Source: CAD feature listing. Evaluate the final solid. Frame: model axes, mm. Face numbers are marked on the shaded views. A direction names the side the tool comes from. Give positions to 0.01 mm unless a question says otherwise; leave off trailing zeros. Write each loop counter-clockwise with the first axis right and the second up, starting at its lowest first coordinate (ties: lowest second). Pieces come first, ordered by that corner, then holes. Notation, with made-up numbers: (36.25, 80) - (95.25, 80) arc R24 cw to (95.25, 93) - close; hole circle Ø3 at (-32.75, 50.5). An arc over 180 degrees is marked (long way). One line per question, with ' | ' between items. Start each with the question number.
(1) Section C-C, the plane x = -2. Return loops of the section in (y, z), plus the area to 3 significant figures.
(2) Section D-D, the plane x = -7.75. Return loops of the section in (y, z).
(3) Ray query, line 1 (X direction, y = -10.1, z = 7.5); line 2 (Y direction, x = -5, z = 10); line 3 (Z direction, x = -8.25, y = -2.75). Return the intervals inside material, ascending. Write a range as [from, to].
(4) Pin query (flat end, axial travel): pin 1 (3 mm diameter, centred on x = 3.5, y = -6, fed in from +Z). Return the tip coordinate at first contact, or that it passes through.
(5) Draft query along Y for the marked faces 1, 2 and 3. Return one class per face: +Y half, -Y half, draft (parallel to the pull), parting line (faces both ways), or undercut.
(6) Section A-A, the plane y = -0.25. Return loops of the section in (x, z).
(7) Section B-B, the plane x = -4.9. Return loops of the section in (y, z).
(8) Access query for the marked faces 4, 5 and 6. Directions: +Z, -Z, +X, -X, +Y, -Y. A direction counts if a zero-diameter tool reaches every point of the face in a straight line with its end or side. Return the directions, or none.
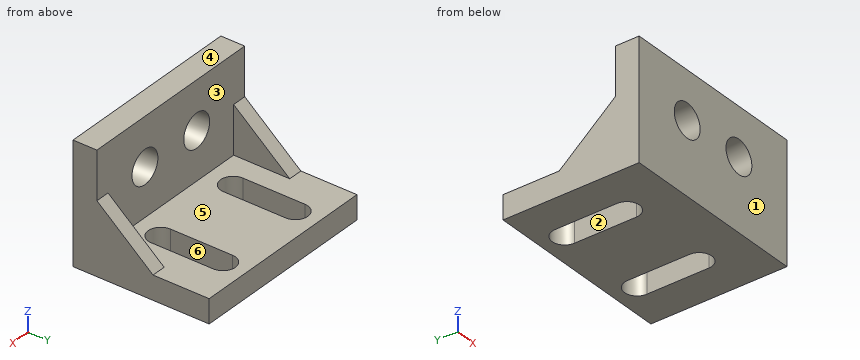
```python
from build123d import *

# Parameters (mm, degrees)
SKETCH1_W           = 20
SKETCH1_H           = 14.251299249
BOSS_EXTRUDE1_DEPTH = 2.5
SKETCH2_W           = 20
SKETCH2_H           = 2.5
BOSS_EXTRUDE2_DEPTH = 10
BOSS_EXTRUDE5_DEPTH = 1.5
SKETCH4_R           = 1.75
CUT_EXTRUDE1_DEPTH  = 20.858072264


with BuildPart() as part:
    # Sketch1 → Boss-Extrude1 (new body)
    with BuildSketch(Plane.XY):
        with Locations((0, -3.814013666)):
            Rectangle(SKETCH1_W, SKETCH1_H)
        with BuildLine():
            Line((-6.210661491, -5.703500897), (-6.210661491, 0.803500897))
            ThreePointArc((-6.210661491, 0.803500897), (-4.9, 2.114162388), (-3.589338509, 0.803500897))
            Line((-3.589338509, 0.803500897), (-3.589338509, -5.703500897))
            ThreePointArc((-3.589338509, -5.703500897), (-4.9, -7.014162388), (-6.210661491, -5.703500897))
        make_face(mode=Mode.SUBTRACT)
        with BuildLine():
            Line((3.589338509, -5.703500897), (3.589338509, 0.803500897))
            ThreePointArc((3.589338509, 0.803500897), (4.9, 2.114162388), (6.210661491, 0.803500897))
            Line((6.210661491, 0.803500897), (6.210661491, -5.703500897))
            ThreePointArc((6.210661491, -5.703500897), (4.9, -7.014162388), (3.589338509, -5.703500897))
        make_face(mode=Mode.SUBTRACT)
    extrude(amount=BOSS_EXTRUDE1_DEPTH)

    # Sketch2 → Boss-Extrude2 (add)
    with BuildSketch(Plane.XY.offset(2.5)):
        with Locations((0, -9.68966329)):
            Rectangle(SKETCH2_W, SKETCH2_H)
    extrude(amount=BOSS_EXTRUDE2_DEPTH)

    # Sketch3 → Boss-Extrude5 (add)
    with BuildSketch(Plane(origin=(10, 0, 0), x_dir=(0, 0, -1), z_dir=(1, 0, 0))):
        Polygon((-7.5, -8.43966329), (-2.5, -2.564013666), (-2.5, -8.43966329), align=None)
    boss_extrude5 = extrude(amount=-BOSS_EXTRUDE5_DEPTH)

    # Sketch4 → Cut-Extrude1 (cut, through all)
    with BuildSketch(Plane(origin=(0, -8.43966329, 0), x_dir=(1, 0, 0), z_dir=(0, 1, 0))):
        with Locations(Location((3.5, -7.5, 0), (0, 0, 270))):
            Circle(SKETCH4_R)
    cut_extrude1 = extrude(amount=-CUT_EXTRUDE1_DEPTH, mode=Mode.SUBTRACT)

    # Mirror1: Boss-Extrude5, Cut-Extrude1 across plane
    add(boss_extrude5.mirror(Plane.ZY))
    add(cut_extrude1.mirror(Plane.ZY), mode=Mode.SUBTRACT)


solid = part.part
```
Check sheet entries:
1) outline: (-10.94, 0) - (3.31, 0) - (3.31, 2.5) - (-8.44, 2.5) - (-8.44, 6.6) - (-10.94, 6.6) - close; (-10.94, 8.4) - (-8.44, 8.4) - (-8.44, 12.5) - (-10.94, 12.5) - close | area: 56.1 mm²
2) outline: (-10.94, 0) - (3.31, 0) - (3.31, 2.5) - (-8.44, 2.5) - (-8.44, 12.5) - (-10.94, 12.5) - close
3) line 1: [-10, -5.25], [-1.75, 1.75], [5.25, 10] | line 2: [-10.94, -8.44] | line 3: [0, 2.5]
4) pin 1: z = 2.5
5) face 1: -Y half | face 2: undercut | face 3: +Y half
6) outline: (-10, 0) - (-6.21, 0) - (-6.21, 2.5) - (-10, 2.5) - close; (-3.59, 0) - (3.59, 0) - (3.59, 2.5) - (-3.59, 2.5) - close; (6.21, 0) - (10, 0) - (10, 2.5) - (6.21, 2.5) - close
7) outline: (-10.94, 0) - (-7.01, 0) - (-7.01, 2.5) - (-8.44, 2.5) - (-8.44, 6.45) - (-10.94, 6.45) - close; (-10.94, 8.55) - (-8.44, 8.55) - (-8.44, 12.5) - (-10.94, 12.5) - close; (2.11, 0) - (3.31, 0) - (3.31, 2.5) - (2.11, 2.5) - close
8) face 4: +Z, +X, -X, +Y, -Y | face 5: +Z, +Y | face 6: +Z, -Z
